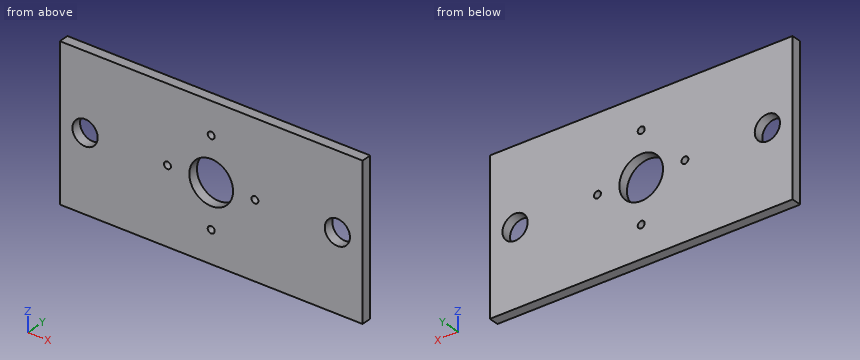
```python
from build123d import *

# Parameters (mm, degrees)
F0_W     = 152.4
F0_H     = 76.2
F0_R     = 1.75
F0_R_2   = 6.35
F0_R_3   = 11
F1_DEPTH = 5


with BuildPart() as f1:
    # F0 (on Front) → F1 (new body)
    with BuildSketch(Plane.XZ):
        Rectangle(F0_W, F0_H)
        with Locations((0, -22)):
            Circle(F0_R, mode=Mode.SUBTRACT)
        with Locations((-63.5, 0)):
            Circle(F0_R_2, mode=Mode.SUBTRACT)
        with Locations((-22, 0)):
            Circle(F0_R, mode=Mode.SUBTRACT)
        Circle(F0_R_3, mode=Mode.SUBTRACT)
        with Locations((22, 0)):
            Circle(F0_R, mode=Mode.SUBTRACT)
        with Locations((63.5, 0)):
            Circle(F0_R_2, mode=Mode.SUBTRACT)
        with Locations((0, 22)):
            Circle(F0_R, mode=Mode.SUBTRACT)
    extrude(amount=F1_DEPTH)


solid = f1.part
```
Source: CAD feature listing. Evaluate the final solid. Frame: model axes, mm. Coordinates: 2 decimals unless noted, no trailing zeros. Write each loop counter-clockwise with the first axis right and the second up, starting at its lowest first coordinate (ties: lowest second). Pieces come first, ordered by that corner, then holes. Notation, with made-up numbers: (54.25, -22.75) -> (100.25, -22.75) arc R19 ccw to (100.25, -9.75) -> close; hole circle Ø11 at (16, -36). An arc over 180 degrees is marked (long way). Return JSON: item names as keys, results as strings. Group by question number.
1) Contact query for a flat-ended pin moving along its axis: P1, Ø2, axis at x = 0, z = 22, coming from the +Y side. Output: stop coordinate, or through.
2) Section query D-D, the plane x = 0. Return loops of the section in (y, z), plus the area to 3 significant figures.
3) Section query B-B, the plane x = 22. Return loops of the section in (y, z), plus the area to 4 significant figures.
4) Section query C-C, the plane z = 22. Return loops of the section in (x, y), plus the area to 4 significant figures.
5) Section query A-A, the plane z = 0. Return loops of the section in (x, y), plus the area to 3 significant figures.
6) Ray query, line 1 along Z through (x, y) = (0, -2.9); line 2 along Z through (x, y) = (-63.5, -2.45); line 3 along Z through (x, y) = (22, -2.5). Return the intervals inside material, ascending.
From the geometry:
{
 "1": {"P1": "through"},
 "2": {"outline": "(-5, -38.1) -> (0, -38.1) -> (0, -23.75) -> (-5, -23.75) -> close; (-5, -20.25) -> (0, -20.25) -> (0, -11) -> (-5, -11) -> close; (-5, 11) -> (0, 11) -> (0, 20.25) -> (-5, 20.25) -> close; (-5, 23.75) -> (0, 23.75) -> (0, 38.1) -> (-5, 38.1) -> close", "area": "236 mm²"},
 "3": {"outline": "(-5, -38.1) -> (0, -38.1) -> (0, -1.75) -> (-5, -1.75) -> close; (-5, 1.75) -> (0, 1.75) -> (0, 38.1) -> (-5, 38.1) -> close", "area": "363.5 mm²"},
 "4": {"outline": "(-76.2, -5) -> (-1.75, -5) -> (-1.75, 0) -> (-76.2, 0) -> close; (1.75, -5) -> (76.2, -5) -> (76.2, 0) -> (1.75, 0) -> close", "area": "744.5 mm²"},
 "5": {"outline": "(-76.2, -5) -> (-69.85, -5) -> (-69.85, 0) -> (-76.2, 0) -> close; (-57.15, -5) -> (-23.75, -5) -> (-23.75, 0) -> (-57.15, 0) -> close; (-20.25, -5) -> (-11, -5) -> (-11, 0) -> (-20.25, 0) -> close; (11, -5) -> (20.25, -5) -> (20.25, 0) -> (11, 0) -> close; (23.75, -5) -> (57.15, -5) -> (57.15, 0) -> (23.75, 0) -> close; (69.85, -5) -> (76.2, -5) -> (76.2, 0) -> (69.85, 0) -> close", "area": "490 mm²"},
 "6": {"line 1": "-38.1 to -23.75, -20.25 to -11, 11 to 20.25, 23.75 to 38.1", "line 2": "-38.1 to -6.35, 6.35 to 38.1", "line 3": "-38.1 to -1.75, 1.75 to 38.1"}
}
